from build123d import *

# Parameters (mm, degrees)
BOSS_EXTRUDE1_DEPTH = 2
SKETCH2_W           = 5
SKETCH2_H           = 25
SKETCH2_W_2         = 20
BOSS_EXTRUDE2_DEPTH = 20
SKETCH3_W           = 25
SKETCH3_H           = 2
BOSS_EXTRUDE3_DEPTH = 25
SKETCH4_W           = 25
SKETCH4_H           = 25
BOSS_EXTRUDE4_DEPTH = 7
BOSS_EXTRUDE5_DEPTH = 5
SKETCH6_W           = 50
SKETCH6_H           = 25
BOSS_EXTRUDE6_DEPTH = 5
BOSS_EXTRUDE7_DEPTH = 30
CUT_EXTRUDE2_DEPTH  = 30
SKETCH10_W          = 5
SKETCH10_H          = 25
CUT_EXTRUDE3_DEPTH  = 20
SKETCH11_W          = 25
SKETCH11_H          = 25
CUT_EXTRUDE4_DEPTH  = 7
SKETCH13_W          = 5
SKETCH13_H          = 25
CUT_EXTRUDE5_DEPTH  = 10
BOSS_EXTRUDE8_REACH = 12
SKETCH14_W          = 10
SKETCH14_H          = 5
SKETCH15_W          = 2.5
SKETCH15_H          = 25
CUT_EXTRUDE6_DEPTH  = 15
SKETCH16_W          = 5
SKETCH16_H          = 15
CUT_EXTRUDE7_DEPTH  = 26
SKETCH17_W          = 5
SKETCH17_H          = 15
CUT_EXTRUDE8_DEPTH  = 43.5
SKETCH18_W          = 5
SKETCH18_H          = 15
CUT_EXTRUDE9_DEPTH  = 6


with BuildPart() as part:
    # Sketch1 → Boss-Extrude1 (new body)
    with BuildSketch(Plane.XY):
        Polygon((-5, 75), (2.5, 25), (2.5, 0), (22.5, 0), (22.5, 25), (30, 75), (30, 100), (25, 100), (25, 75), (0, 75), (0, 100), (-5, 100), align=None)
    extrude(amount=BOSS_EXTRUDE1_DEPTH)

    # Sketch2 → Boss-Extrude2 (add)
    with BuildSketch(Plane(origin=(0, 0, 0), x_dir=(-1, 0, 0), z_dir=(0, 0, -1))):
        with Locations((-27.5, 87.5)):
            Rectangle(SKETCH2_W, SKETCH2_H)
        with Locations((2.5, 87.5)):
            Rectangle(SKETCH2_W, SKETCH2_H)
        with Locations((-12.5, 12.5)):
            Rectangle(SKETCH2_W_2, SKETCH2_H)
    extrude(amount=BOSS_EXTRUDE2_DEPTH)

    # Sketch3 → Boss-Extrude3 (add)
    with BuildSketch(Plane(origin=(0, 75, 0), x_dir=(1, 0, 0), z_dir=(0, 1, 0))):
        with Locations((12.5, -1)):
            Rectangle(SKETCH3_W, SKETCH3_H)
    extrude(amount=BOSS_EXTRUDE3_DEPTH)

    # Sketch4 → Boss-Extrude4 (add)
    with BuildSketch(Plane(origin=(0, 0, 0), x_dir=(-1, 0, 0), z_dir=(0, 0, -1))):
        with Locations((-12.5, 87.5)):
            Rectangle(SKETCH4_W, SKETCH4_H)
    extrude(amount=BOSS_EXTRUDE4_DEPTH)

    # Sketch5 → Boss-Extrude5 (add)
    with BuildSketch(Plane(origin=(0, 0, 0), x_dir=(-1, 0, 0), z_dir=(0, 0, -1))):
        Polygon((5, 75), (5, 0), (-2.5, 0), (-22.5, 0), (-30, 0), (-30, 75), (-30, 100), (5, 100), align=None)
    extrude(amount=-BOSS_EXTRUDE5_DEPTH)

    # Sketch6 → Boss-Extrude6 (add)
    with BuildSketch(Plane.XY.offset(5)):
        with Locations((12.5, 12.5)):
            Rectangle(SKETCH6_W, SKETCH6_H)
    extrude(amount=-BOSS_EXTRUDE6_DEPTH)

    # Sketch8 → Boss-Extrude7 (add)
    with BuildSketch(Plane.XZ.offset(-75)):
        Polygon((-5, 0), (-5, -20), (0, -20), (0, -7), (25, -7), (25, -20), (30, -20), (30, 0), align=None)
    extrude(amount=BOSS_EXTRUDE7_DEPTH)

    # Sketch9 → Cut-Extrude2 (cut)
    with BuildSketch(Plane(origin=(0, 100, 0), x_dir=(1, 0, 0), z_dir=(0, 1, 0))):
        Polygon((30, 20), (25, 20), (25, 7), (0, 7), (0, 20), (-5, 20), (-5, -5), (30, -5), align=None)
    extrude(amount=-CUT_EXTRUDE2_DEPTH, mode=Mode.SUBTRACT)

    # Sketch10 → Cut-Extrude3 (cut)
    with BuildSketch(Plane(origin=(0, 0, -20), x_dir=(-1, 0, 0), z_dir=(0, 0, -1))):
        with Locations((-20, 12.5)):
            Rectangle(SKETCH10_W, SKETCH10_H)
        with Locations((-5, 12.5)):
            Rectangle(SKETCH10_W, SKETCH10_H)
    extrude(amount=-CUT_EXTRUDE3_DEPTH, mode=Mode.SUBTRACT)

    # Sketch11 → Cut-Extrude4 (cut)
    with BuildSketch(Plane(origin=(0, 0, -7), x_dir=(-1, 0, 0), z_dir=(0, 0, -1))):
        with Locations((-12.5, 57.5)):
            Rectangle(SKETCH11_W, SKETCH11_H)
    extrude(amount=-CUT_EXTRUDE4_DEPTH, mode=Mode.SUBTRACT)

    # Sketch13 → Cut-Extrude5 (cut)
    with BuildSketch(Plane(origin=(17.5, 0, 0), x_dir=(0, 0, -1), z_dir=(1, 0, 0))):
        Polygon((5, 25), (5, 20), (10, 20), (10, 5), (0, 5), (0, 25), align=None)
        with Locations((17.5, 12.5)):
            Rectangle(SKETCH13_W, SKETCH13_H)
    extrude(amount=-CUT_EXTRUDE5_DEPTH, mode=Mode.SUBTRACT)

    # Sketch14 → Boss-Extrude8 (add, up to next)
    with BuildSketch(Plane.XY.offset(-5), mode=Mode.PRIVATE) as boss_extrude8_sk1:
        with Locations((12.5, 22.5)):
            Rectangle(SKETCH14_W, SKETCH14_H)
    boss_extrude8_tool1 = extrude(boss_extrude8_sk1.sketch, amount=BOSS_EXTRUDE8_REACH, mode=Mode.PRIVATE) - part.part
    add(boss_extrude8_tool1.solids().sort_by_distance((12.5, 22.5, -5))[0])

    # Sketch15 → Cut-Extrude6 (cut)
    with BuildSketch(Plane(origin=(0, 0, -15), x_dir=(-1, 0, 0), z_dir=(0, 0, -1))):
        with Locations((-8.75, 12.5)):
            Rectangle(SKETCH15_W, SKETCH15_H)
        with Locations((-16.25, 12.5)):
            Rectangle(SKETCH15_W, SKETCH15_H)
    extrude(amount=-CUT_EXTRUDE6_DEPTH, mode=Mode.SUBTRACT)

    # Sketch16 → Cut-Extrude7 (cut, through all)
    with BuildSketch(Plane.XY.offset(5)):
        with Locations((-5, 12.5)):
            Rectangle(SKETCH16_W, SKETCH16_H)
        with Locations((30, 12.5)):
            Rectangle(SKETCH16_W, SKETCH16_H)
    extrude(amount=-CUT_EXTRUDE7_DEPTH, mode=Mode.SUBTRACT)

    # Sketch17 → Cut-Extrude8 (cut, through all)
    with BuildSketch(Plane(origin=(30, 0, 0), x_dir=(0, 0, -1), z_dir=(1, 0, 0))):
        with Locations((2.5, 57.5)):
            Rectangle(SKETCH17_W, SKETCH17_H)
    extrude(amount=-CUT_EXTRUDE8_DEPTH, mode=Mode.SUBTRACT)

    # Sketch18 → Cut-Extrude9 (cut, through all)
    with BuildSketch(Plane(origin=(0, 0, 0), x_dir=(-1, 0, 0), z_dir=(0, 0, -1))):
        with Locations((-2.5, 57.5)):
            Rectangle(SKETCH18_W, SKETCH18_H)
        with Locations((-22.5, 57.5)):
            Rectangle(SKETCH18_W, SKETCH18_H)
    extrude(amount=-CUT_EXTRUDE9_DEPTH, mode=Mode.SUBTRACT)


solid = part.part
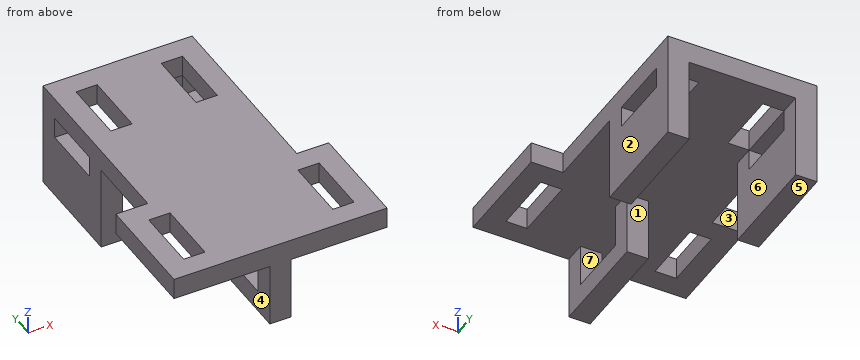
Could you check a few things on this model? Use its own coordinates, in mm. Face numbers are marked on the shaded views. A direction names the side the tool comes from. Give positions to 0.01 mm unless a question says otherwise; leave off trailing zeros. Loops run counter-clockwise (first coordinate to the right, second up) from the corner with the lowest first, then second, coordinate; pieces in that order, holes last. Notation, with made-up numbers: (48.25, -6) -> (97.25, -6) arc R15 cw to (97.25, 8) -> close; hole circle Ø6 at (55, 0.5). An arc over 180 degrees is marked (long way). Return JSON: item names as keys, results as strings.
Item 1: If we section it at C-C on x = 2: List the corners of the cut face in (y, z) for me.
Geometry results:
{"outline": "(0, 0) -> (50, 0) -> (50, 5) -> (0, 5) -> close; (65, 0) -> (70, 0) -> (70, 5) -> (65, 5) -> close"}
Item 2: We'd pull the mould along Z, two halves only. Please class the marked faces 5, 6 and 7: +Z half, -Z half, draft (parallel to the pull), parting line (faces both ways), or undercut.
Geometry results:
{"face 5": "-Z half", "face 6": "draft", "face 7": "undercut"}
Item 3: If we section it at D-D on z = -12.25: List the corners of the cut face in (x, y) for me, plus the area to 3 significant figures.
Geometry results:
{"outline": "(-5, 45) -> (0, 45) -> (0, 70) -> (-5, 70) -> close; (10, 0) -> (15, 0) -> (15, 25) -> (10, 25) -> close; (25, 45) -> (30, 45) -> (30, 70) -> (25, 70) -> close", "area": "375 mm²"}
Item 4: I'm going to push flat-ended pins straight in: pin 1 (3 mm diameter, centred on x = 12, y = 40.5, fed in from -Z); pin 2 (1.5 mm diameter, centred on x = 32.5, z = 2, fed in from +Y); pin 3 (12 mm diameter, centred on y = 14, z = -7.5, fed in from +X); pin 4 (10 mm diameter, centred on y = 32.5, z = -15, fed in from -X). Where does each tip first touch, or does it pass through?
Geometry results:
{"pin 1": "stops at z = 0", "pin 2": "stops at y = 25", "pin 3": "stops at x = 15", "pin 4": "passes through"}
Item 5: I need wall thicknesses on L1, parallel to X at y = 59.5, z = -7.75; L2, parallel to Y at x = 23, z = 3; L3, parallel to Z at x = 23, y = 37. Which ranges of each line are inside material? Lowest first, please. Write a range as from..to.
Geometry results:
{"L1": "x = -5..0, 25..30", "L2": "y = 0..50, 65..70", "L3": "z = 0..5"}
Item 6: Which directions (+Z, -Z, +X, -X, +Y, -Y) give clear straight access to the entire face, cutting with the end or side of a thin tool? Please do the marked faces 1, 2, 3 and 4.
Geometry results:
{"face 1": "-Z, +X, -X, +Y", "face 2": "+Z, -Z, +X, +Y", "face 3": "+Z, -Z, -X, +Y", "face 4": "-Z, -X, +Y, -Y"}
Item 7: If we section it at A-A on z = -18.25: List the corners of the cut face in (x, y) for me, plus the area to 3 significant figures.
Geometry results:
{"outline": "(-5, 45) -> (0, 45) -> (0, 70) -> (-5, 70) -> close; (25, 45) -> (30, 45) -> (30, 70) -> (25, 70) -> close", "area": "250 mm²"}
Item 8: If we section it at B-B on y = 52.5: List the corners of the cut face in (x, z) for me.
Geometry results:
{"outline": "(-5, -20) -> (0, -20) -> (0, -5) -> (-5, -5) -> close; (-5, 0) -> (0, 0) -> (0, 5) -> (-5, 5) -> close; (5, 0) -> (20, 0) -> (20, 5) -> (5, 5) -> close; (25, -20) -> (30, -20) -> (30, -5) -> (25, -5) -> close; (25, 0) -> (30, 0) -> (30, 5) -> (25, 5) -> close"}
